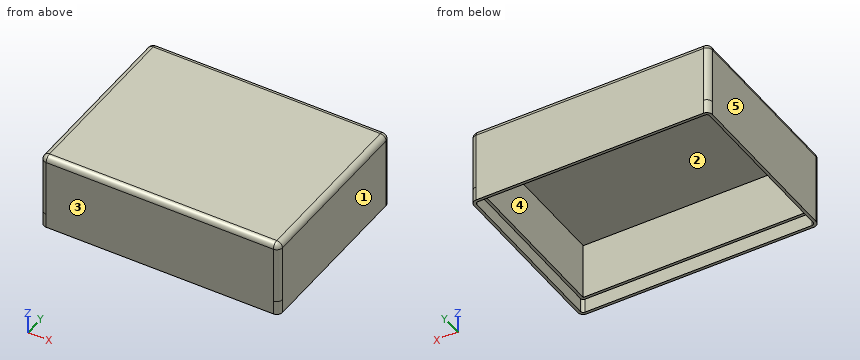
```python
from build123d import *

# Parameters (mm, degrees)
BOX001_W       = 80
BOX001_H       = 60
BOX001_DEPTH   = 20
THICKNESS001_T = 2
PAD001_DEPTH   = 5


with BuildPart() as part:
    # Box001 → Box001 (new body)
    with BuildSketch(Plane.XY.offset(10)):
        with Locations((40, 30)):
            Rectangle(BOX001_W, BOX001_H)
    extrude(amount=BOX001_DEPTH)

    # Thickness001
    thickness001_openings = [part.faces().sort_by_distance(p)[0] for p in [
        (40, 30, 10),
    ]]
    offset(amount=THICKNESS001_T, openings=thickness001_openings)

    # Sketch005 → Pad001 (new body)
    with BuildSketch(Plane(origin=(0, 0, 10), x_dir=(1, 0, 0), z_dir=(0, 0, -1))):
        with BuildLine():
            Line((0, 2), (80, 2))
            ThreePointArc((82, 0), (81.414214, 1.414214), (80, 2))
            Line((82, 0), (82, -60))
            ThreePointArc((80, -62), (81.414214, -61.414214), (82, -60))
            Line((80, -62), (0, -62))
            ThreePointArc((-2, -60), (-1.414214, -61.414214), (0, -62))
            Line((-2, -60), (-2, 0))
            ThreePointArc((0, 2), (-1.414214, 1.414214), (-2, 0))
        make_face()
        with BuildLine():
            Line((0, 1), (80, 1))
            ThreePointArc((81, 0), (80.707107, 0.707107), (80, 1))
            Line((81, 0), (81, -60))
            ThreePointArc((80, -61), (80.707107, -60.707107), (81, -60))
            Line((80, -61), (0, -61))
            ThreePointArc((-1, -60), (-0.707107, -60.707107), (0, -61))
            Line((-1, -60), (-1, 0))
            ThreePointArc((0, 1), (-0.707107, 0.707107), (-1, 0))
        make_face(mode=Mode.SUBTRACT)
    extrude(amount=PAD001_DEPTH)


solid = part.part
```
For this review, take the finished solid that the model builds, in its own axes (mm). Face numbers are marked on the shaded views. A direction names the side the tool comes from. Round coordinates to 2 decimals unless told otherwise and drop trailing zeros. Write each loop counter-clockwise with the first axis right and the second up, starting at its lowest first coordinate (ties: lowest second). Pieces come first, ordered by that corner, then holes. Notation, with made-up numbers: (59, 26.25) - (88, 26.25) arc R27 cw to (88, 60.25) - close; hole circle Ø10 at (80.5, -19). An arc over 180 degrees is marked (long way). Put each result on its own line as item: value.
Q1. Wall thickness on probe 1 along X at (y, z) = (50, 14.75); probe 2 along Y at (x, z) = (22.5, 20.25); probe 3 along Y at (x, z) = (7.5, 7.5): over which ranges is each line inside the solid? List them lowest first.
Solved:
probe 1: x = -2 to 0, 80 to 82
probe 2: y = -2 to 0, 60 to 62
probe 3: y = -2 to -1, 61 to 62
Q2. Machinability: for the marked faces 4 and 5, which of the approach directions +Z, -Z, +X, -X, +Y, -Y give a long, thin tool a straight path to every point of the face, cutting with its end or side? Answer none if there is none.
Solved:
face 4: -Z
face 5: +Z, -Z, -X, +Y, -Y
Q3. We need section D-D (z = 8.75). Give the boundary of the cut face in (x, y).
Solved:
outline: (-2, 0) arc R2 ccw to (0, -2) - (80, -2) arc R2 ccw to (82, 0) - (82, 60) arc R2 ccw to (80, 62) - (0, 62) arc R2 ccw to (-2, 60) - close; hole (-1, 0) arc R1 ccw to (0, -1) - (80, -1) arc R1 ccw to (81, 0) - (81, 60) arc R1 ccw to (80, 61) - (0, 61) arc R1 ccw to (-1, 60) - close
Q4. Mouldability with a two-part tool opening along X and no side actions: class the marked faces 1, 2 and 3 as released by +X, released by -X, zero draft, split by the parting line, or undercut.
Solved:
face 1: released by +X
face 2: undercut
face 3: zero draft
Q5. We need section C-C (y = 56). Give the boundary of the cut face in (x, z).
Solved:
outline: (-2, 5) - (-1, 5) - (-1, 10) - (0, 10) - (0, 30) - (80, 30) - (80, 10) - (81, 10) - (81, 5) - (82, 5) - (82, 30) arc R2 ccw to (80, 32) - (0, 32) arc R2 ccw to (-2, 30) - close
Q6. We need section B-B (x = 19.5). Give the boundary of the cut face in (y, z).
Solved:
outline: (-2, 5) - (-1, 5) - (-1, 10) - (0, 10) - (0, 30) - (60, 30) - (60, 10) - (61, 10) - (61, 5) - (62, 5) - (62, 30) arc R2 ccw to (60, 32) - (0, 32) arc R2 ccw to (-2, 30) - close
Q7. Insertion check: pin 1 Ø2 at (x, y) = (57, 17) entering from -Z. The pin has a flat end and moves straight along its axis. Give the tip position at first contact, or say it passes through.
Solved:
pin 1: stops at z = 30
Q8. We need section A-A (z = 15.5). Give the boundary of the cut face in (x, y).
Solved:
outline: (-2, 0) arc R2 ccw to (0, -2) - (80, -2) arc R2 ccw to (82, 0) - (82, 60) arc R2 ccw to (80, 62) - (0, 62) arc R2 ccw to (-2, 60) - close; hole (0, 0) - (80, 0) - (80, 60) - (0, 60) - close
